For this review, take the finished solid that the model builds, in its own axes (mm). A direction names the side the tool comes from. Round coordinates to 2 decimals unless told otherwise and drop trailing zeros. Loops run counter-clockwise (first coordinate to the right, second up) from the corner with the lowest first, then second, coordinate; pieces in that order, holes last.
1) Wall thickness on L1, parallel to Y at x = 0.75, z = 8 (3 decimals); L2, parallel to Z at x = 1, y = 5.25; L3, parallel to Z at x = -1.5, y = 11.75: over which ranges is each line inside the solid? List them lowest first.
2) Take a section at A-A (z = 16.5). State the section outline as (x, y) points (3 decimals), then the cut area to 3 significant figures.
3) Insertion check: pin 1 (1 mm diameter, centred on x = 0, z = 17, fed in from +Y) (3 decimals); pin 2 (6 mm diameter, centred on y = 4.5, z = -13, fed in from -X); pin 3 (3 mm diameter, centred on x = 0, y = 6.5, fed in from -Z). Each pin has a flat end and moves straight along its axis. Give the tip position at first contact, or say it passes through.
4) Tool access review of faces 1 (the flat face through (-1.598, 2.744, -13.383)), 2 (the flat face through (0, 3.175, 14)), 3 (the flat face through (-1.598, 2.744, 13.042)): name each direction out of +Z, -Z, +X, -X, +Y, -Y from which nothing blocks a thin tool from reaching the whole face with its end or side.
5) Take a section at B-B (y = 4.5). State the section outline as (x, z) points, then the cut area to 3 significant figures.
Autodesk Inventor part; units mm, degrees
ref_plane "YZ Plane" through (0, 0, 0) normal (1, 0, 0) x (0, 1, 0)
ref_plane "XZ Plane" through (0, 0, 0) normal (0, 1, 0) x (-1, 0, 0)
ref_plane "XY Plane" through (0, 0, 0) normal (0, 0, 1) x (1, 0, 0)
sketch "Sketch1" plane through (0, 0, 0) normal (0, 0, 1) x (1, 0, 0)
  line L0 (3.175, 0.8507) -> (3.175, -0.8507)
  line L1 (3.175, -0.8507) -> (2.3243, -2.3243)
  line L2 (2.3243, -2.3243) -> (0.8507, -3.175)
  line L3 (0.8507, -3.175) -> (-0.8507, -3.175)
  line L4 (-0.8507, -3.175) -> (-2.3243, -2.3243)
  line L5 (-2.3243, -2.3243) -> (-3.175, -0.8507)
  line L6 (-3.175, -0.8507) -> (-3.175, 0.8507)
  line L7 (-3.175, 0.8507) -> (-2.3243, 2.3243)
  line L8 (-2.3243, 2.3243) -> (-0.8507, 3.175)
  line L9 (-0.8507, 3.175) -> (0.8507, 3.175)
  line L10 (0.8507, 3.175) -> (2.3243, 2.3243)
  line L11 (2.3243, 2.3243) -> (3.175, 0.8507)
  line L12 (0, 0) -> (0, 3.175) construction
  dimension "d9" = 6.35
extrude "Extrusion1" add sketch "Sketch1" along normal blind 25.4 and the other way blind 25.4
sketch "Sketch2" plane through (0, 0, 0) normal (0, 1, 0) x (-1, 0, 0)
  circle A0 centre (0, 0) radius 2.54
  dimension "diamCamSlot" = 5.08
extrude "Extrusion2" add sketch "Sketch2" along normal blind 12.7
fillet "Fillet1" radius 1.5875 1 edges at (2.54, 12.7, 0)
equation "\"d9\" = camDiam"
equation "\"camDiam\" = 6.35"
properties part number "vexCamPost11"
Response:
1. L1: y = -3.175 to 3.175
1. L2: z = -2.33 to 2.33
1. L3: z = -1.88 to 1.88
2. outline: (-3.175, -0.851) - (-2.324, -2.324) - (-0.851, -3.175) - (0.851, -3.175) - (2.324, -2.324) - (3.175, -0.851) - (3.175, 0.851) - (2.324, 2.324) - (0.851, 3.175) - (-0.851, 3.175) - (-2.324, 2.324) - (-3.175, 0.851) - close
2. area: 32.4 mm2
3. pin 1: stops at y = 3.175
3. pin 2: stops at x = -2.8
3. pin 3: stops at z = -2.54
4. face 1: -Z, -X, +Y
4. face 2: +Z, +X, -X, +Y
4. face 3: +Z, -X, +Y
5. outline: circle Ø5.08 at (0, 0)
5. area: 20.3 mm2
